Input: part model. Units: mm. Frame: model coordinates. Coordinates: 2 decimals unless noted, no trailing zeros. Order: outer loops, then holes, each group sorted by start corner. A loop starts at its lowest first (then second) coordinate and runs counter-clockwise, first axis right, second up.
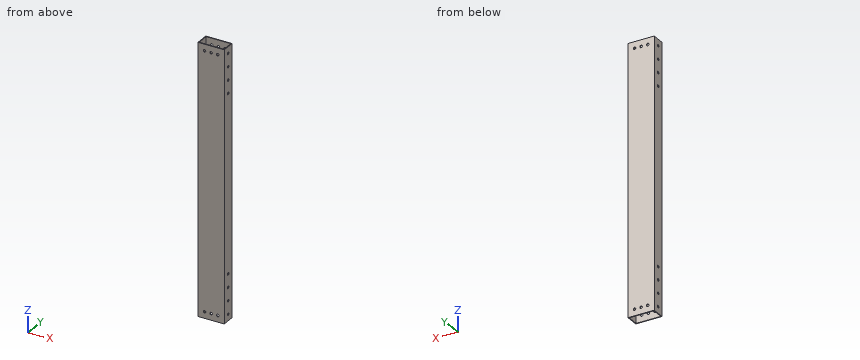
from build123d import *

# Parameters (mm, degrees)
SKETCH1_W           = 50.8
SKETCH1_H           = 25.4
SKETCH1_W_2         = 47.625
SKETCH1_H_2         = 22.225
BOSS_EXTRUDE1_DEPTH = 260.35
SKETCH2_R           = 2.4892
CUT_EXTRUDE1_DEPTH  = 263.8163665
SKETCH3_R           = 2.4892
CUT_EXTRUDE2_DEPTH  = 266.563650562


with BuildPart() as part:
    # Sketch1 → Boss-Extrude1 (new, symmetric)
    with BuildSketch(Plane.XY):
        Rectangle(SKETCH1_W, SKETCH1_H)
        Rectangle(SKETCH1_W_2, SKETCH1_H_2, mode=Mode.SUBTRACT)
    extrude(amount=BOSS_EXTRUDE1_DEPTH, both=True)

    # Sketch2 → Cut-Extrude1 (cut, through all)
    with BuildSketch(Plane(origin=(0, 12.7, 0), x_dir=(1, 0, 0), z_dir=(0, 1, 0))):
        with Locations(Location((-12.7, 247.65, 0), (0, 0, 270))):
            Circle(SKETCH2_R)
        with Locations(Location((0, 247.65, 0), (0, 0, 270))):
            Circle(SKETCH2_R)
        with Locations(Location((12.7, 247.65, 0), (0, 0, 270))):
            Circle(SKETCH2_R)
        with Locations((12.7, -247.65)):
            Circle(SKETCH2_R)
        with Locations((0, -247.65)):
            Circle(SKETCH2_R)
        with Locations((-12.7, -247.65)):
            Circle(SKETCH2_R)
    extrude(amount=-CUT_EXTRUDE1_DEPTH, mode=Mode.SUBTRACT)

    # Sketch3 → Cut-Extrude2 (cut, through all)
    with BuildSketch(Plane(origin=(25.4, 0, 0), x_dir=(0, 0, -1), z_dir=(1, 0, 0))):
        with Locations((247.65, 0)):
            Circle(SKETCH3_R)
        with Locations(Location((-247.65, 0, 0), (0, 0, 180))):
            Circle(SKETCH3_R)
        with Locations((222.25, 0)):
            Circle(SKETCH3_R)
        with Locations((196.85, 0)):
            Circle(SKETCH3_R)
        with Locations((171.45, 0)):
            Circle(SKETCH3_R)
        with Locations(Location((-171.45, 0, 0), (0, 0, 180))):
            Circle(SKETCH3_R)
        with Locations(Location((-196.85, 0, 0), (0, 0, 180))):
            Circle(SKETCH3_R)
        with Locations(Location((-222.25, 0, 0), (0, 0, 180))):
            Circle(SKETCH3_R)
    extrude(amount=-CUT_EXTRUDE2_DEPTH, mode=Mode.SUBTRACT)


solid = part.part
Item 1: Ray query, probe 1 along X at (y, z) = (12.3, -247.65); probe 2 along X at (y, z) = (-7.25, 108); probe 3 along Y at (x, z) = (14, -73). Return the intervals inside material, ascending.
Response values:
probe 1: x = -25.4 to -15.19, -10.21 to -2.49, 2.49 to 10.21, 15.19 to 25.4
probe 2: x = -25.4 to -23.81, 23.81 to 25.4
probe 3: y = -12.7 to -11.11, 11.11 to 12.7
Item 2: Pin query (flat end, axial travel): pin 1 Ø4 at (y, z) = (0, 222.25) entering from -X (3 decimals). Return the tip coordinate at first contact, or that it passes through.
Response values:
pin 1: passes through
Item 3: Cut plane A-A on z = -27. Return loops of the section in (x, y), then the cut area to 3 significant figures.
Response values:
outline: (-25.4, -12.7) - (25.4, -12.7) - (25.4, 12.7) - (-25.4, 12.7) - close; hole (-23.81, -11.11) - (23.81, -11.11) - (23.81, 11.11) - (-23.81, 11.11) - close
area: 232 mm2
